from build123d import *

# Parameters (mm, degrees)
F0_W     = 30
F0_H     = 10
F1_DEPTH = 5
F0_W_2   = 10
F0_H_2   = 30
F2_DEPTH = 25


with BuildPart() as f1:
    # F0 (on Top) → F1 (new body)
    with BuildSketch(Plane.XY):
        with Locations((-25, 35)):
            Rectangle(F0_W, F0_H)
    extrude(amount=F1_DEPTH)



with BuildPart() as f1b:
    # F0 (on Top) → F1, piece 2 (new body)
    with BuildSketch(Plane.XY):
        with Locations((-5, 15)):
            Rectangle(F0_W_2, F0_H_2)
    extrude(amount=F1_DEPTH)


with BuildPart() as f1_1:
    add(f1.part)

    add(f1b.part)  # F2 merges F1b
    # F0 (on Top) → F2 (join)
    with BuildSketch(Plane.XY):
        Polygon((-14, 0), (-10, 0), (-10, 30), (-40, 30), (-40, 26), (-14, 26), align=None)
    extrude(amount=F2_DEPTH)


solid = f1_1.part
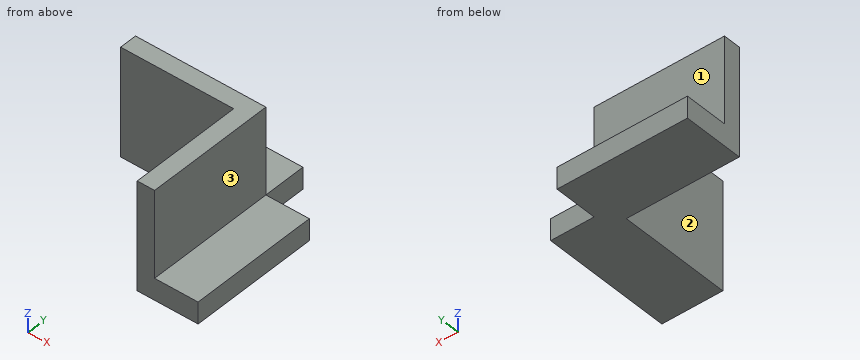
Input: part model. Units: mm. Frame: model coordinates. Face numbers are marked on the shaded views. A direction names the side the tool comes from. Coordinates: 2 decimals unless noted, no trailing zeros. Loops run counter-clockwise (first coordinate to the right, second up) from the corner with the lowest first, then second, coordinate; pieces in that order, holes last. Notation, with made-up numbers: (29, 39) -> (80, 39) arc R19 cw to (80, 75) -> close; hole circle Ø9 at (-26.5, 19). An arc over 180 degrees is marked (long way). Write item = value, one per line. Start each with the question number.
Item 1: Cut plane A-A, the plane z = 3.75. Return loops of the section in (x, y).
Item 2: Cut plane C-C, the plane x = -5. Return loops of the section in (y, z), plus the area to 3 significant figures.
Item 3: Material intervals for line 1 (Y direction, x = -22, z = 3); line 2 (Y direction, x = -19, z = 22.25); line 3 (X direction, y = 18.5, z = 5.75), sorted ascending.
Item 4: Cut plane B-B, the plane y = 11. Return loops of the section in (x, z), plus the area to 3 significant figures.
Item 5: Cut plane D-D, the plane y = 28. Return loops of the section in (x, z).
Item 6: Reachability of the marked faces 1, 2 and 3 from +Z, -Z, +X, -X, +Y, -Y: full face, straight path, thin tool, end or side. Return the list, or none.
Item 7: First-contact query: P1, Ø5.5, axis at y = 36.5, z = 2, coming from the +X side; P2, Ø2, axis at y = 8, z = 17, coming from the -X side; P3, Ø12, axis at y = 17, z = 4.5, coming from the +X side; P4, Ø7.5, axis at x = -29, z = 11, coming from the -Y side. Flat tips, straight axial feed; report the tip coordinate or a pass-through.
Ans:
q1.outline = (-40, 26) -> (-14, 26) -> (-14, 0) -> (0, 0) -> (0, 30) -> (-10, 30) -> (-10, 40) -> (-40, 40) -> close
q2.outline = (0, 0) -> (30, 0) -> (30, 5) -> (0, 5) -> close
q2.area = 150 mm²
q3.line_1 = 26 to 40
q3.line_2 = 26 to 30
q3.line_3 = -14 to -10
q4.outline = (-14, 0) -> (0, 0) -> (0, 5) -> (-10, 5) -> (-10, 25) -> (-14, 25) -> close
q4.area = 150 mm²
q5.outline = (-40, 0) -> (0, 0) -> (0, 5) -> (-10, 5) -> (-10, 25) -> (-40, 25) -> close
q6.face_1 = +Z, +X, -X, +Y
q6.face_2 = +Z, -Z, -X, -Y
q6.face_3 = +Z, +X, +Y, -Y
q7.P1 = -10
q7.P2 = -14
q7.P3 = 0
q7.P4 = 26
